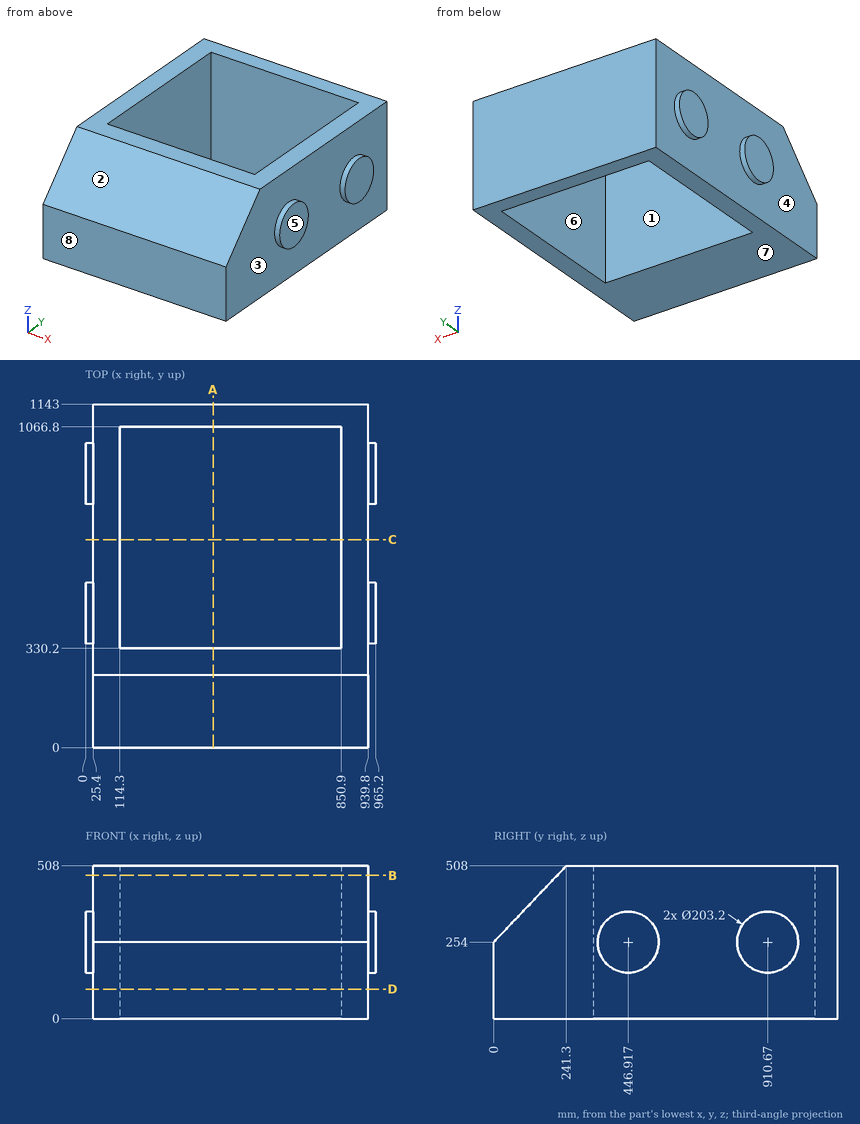
Design review of the part shown in the three views and the two pictorial views. Dimensions are in mm from the part's minimum x, y and z. A direction names the side the tool comes from. Round coordinates to 2 decimals unless told otherwise and drop trailing zeros. Loops run counter-clockwise (first coordinate to the right, second up) from the corner with the lowest first, then second, coordinate; pieces in that order, holes last. Notation, with made-up numbers: (51.5, -12) - (63.5, -12) arc R28 ccw to (63.5, 11) - close; hole circle Ø8 at (-27.75, 71.25). An arc over 180 degrees is marked (long way). One line per item, written item: value. Start each with the question number.
Item 1: Clearance check with flat-ended pins moving along their axes: pin 1 Ø2 at (y, z) = (533, 69.5) entering from -X; pin 2 Ø1 at (y, z) = (226, 110.5) entering from +X. State where each tip first meets the part, or that it passes through.
Item 2: Take a section at A-A (x = 424). Give the boundary of the cut face in (y, z), plus the area to 3 significant figures.
Item 3: Take a section at D-D (z = 97.5). Give the boundary of the cut face in (x, y), plus the area to 3 significant figures.
Item 4: Take a section at B-B (z = 476). Give the boundary of the cut face in (x, y).
Item 5: The part is to be moulded in two halves that separate along Y. For the marked faces 6, 7 and 8, say which applies: +Y half, -Y half, draft (parallel to the pull), parting line (faces both ways), or undercut.
Item 6: Take a section at C-C (y = 692). Give the boundary of the cut face in (x, z), plus the area to 3 significant figures.
Item 7: For the marked faces 1, 2, 3, 4 and 5, list the 3-axis set-ups (+Z, -Z, +X, -X, +Y, -Y) from which the entire face can be reached by the end or side of a thin tool; tool diameter is ignored.
Item 8: For L1, parallel to Y at x = 519, z = 136.5; L2, parallel to X at y = 915.5, z = 21; L3, parallel to Y at x = 262, z = 374, list the stretches that pass through material, from the lowest coordinate up.
Answer below:
1. pin 1: stops at x = 25.4
1. pin 2: stops at x = 939.8
2. outline: (0, 0) - (330.2, 0) - (330.2, 508) - (241.3, 508) - (0, 254) - close; (1066.8, 0) - (1143, 0) - (1143, 508) - (1066.8, 508) - close
2. area: 176,000 mm2
3. outline: (25.4, 0) - (939.8, 0) - (939.8, 1143) - (25.4, 1143) - close; hole (114.3, 330.2) - (850.9, 330.2) - (850.9, 1066.8) - (114.3, 1066.8) - close
3. area: 503,000 mm2
4. outline: (25.4, 210.9) - (939.8, 210.9) - (939.8, 1143) - (25.4, 1143) - close; hole (114.3, 330.2) - (850.9, 330.2) - (850.9, 1066.8) - (114.3, 1066.8) - close
5. face 6: undercut
5. face 7: draft
5. face 8: -Y half
6. outline: (25.4, 0) - (114.3, 0) - (114.3, 508) - (25.4, 508) - close; (850.9, 0) - (939.8, 0) - (939.8, 508) - (850.9, 508) - close
6. area: 90,300 mm2
7. face 1: +Z, -Z
7. face 2: +Z, +X, -X, -Y
7. face 3: +X
7. face 4: -X
7. face 5: +Z, -Z, +X, +Y, -Y
8. L1: y = 0 to 330.2, 1066.8 to 1143
8. L2: x = 25.4 to 114.3, 850.9 to 939.8
8. L3: y = 114 to 330.2, 1066.8 to 1143
